Part model, mm, in its own coordinate system. Face numbers are marked on the shaded views. Round coordinates to 2 decimals unless told otherwise and drop trailing zeros. Loops run counter-clockwise (first coordinate to the right, second up) from the corner with the lowest first, then second, coordinate; pieces in that order, holes last. Notation, with made-up numbers: (-39.5, 35.25) -> (13.5, 35.25) arc R4 ccw to (13.5, 41.25) -> close; hole circle Ø6 at (66.25, 44). An arc over 180 degrees is marked (long way). Answer as CSV lines item,"result".
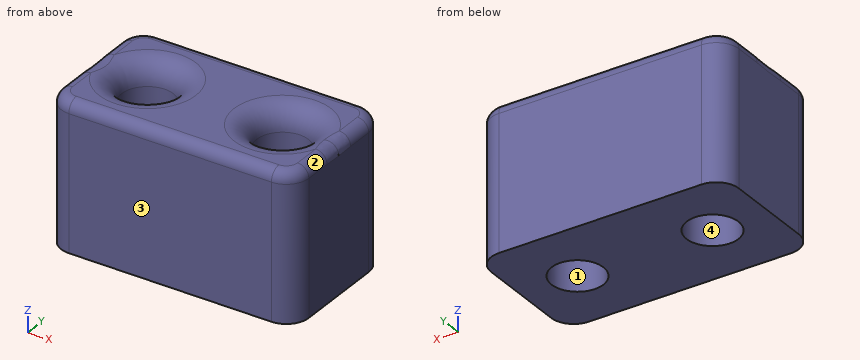
Autodesk Inventor part; units mm, degrees
ref_plane "YZ Plane" through (0, 0, 0) normal (1, 0, 0) x (0, 1, 0)
ref_plane "XZ Plane" through (0, 0, 0) normal (0, 1, 0) x (-1, 0, 0)
ref_plane "XY Plane" through (0, 0, 0) normal (0, 0, 1) x (1, 0, 0)
sketch "Sketch1" plane through (0, 0, 0) normal (0, 0, 1) x (1, 0, 0)
  line L0 (-11, -6) -> (11, -6)
  line L1 (11, -6) -> (11, 6)
  line L2 (11, 6) -> (-11, 6)
  line L3 (-11, 6) -> (-11, -6)
  line L4 (-11, -6) -> (11, 6) construction
  line L5 (11, -6) -> (-11, 6) construction
  circle A0 centre (-6, 0) radius 2.3
  circle A1 centre (6, 0) radius 2.3
  line L6 (-6, 0) -> (0, 0) construction
  line L7 (0, 0) -> (6, 0) construction
  dimension "d0" = 12
  dimension "d1" = 4.6
  dimension "d2" = 12
  dimension "d3" = 5
extrude "Extrusion1" add sketch "Sketch1" along normal blind 13
fillet "Fillet1" radius 2 6 edges at (11, 6, 6.5) (11, -6, 6.5) (-11, 6, 6.5) (-11, -6, 6.5) (-8.3, 0, 13) (3.7, 0, 13)
fillet "Fillet2" radius 1 8 edges at (-10.4142, 5.4142, 13) (-11, 0, 13) (-10.4142, -5.4142, 13) (0, -6, 13) (10.4142, -5.4142, 13) (11, 0, 13) (10.4142, 5.4142, 13) (0, 6, 13)
properties part number "spacer"
Q1. Two-plate mould, pull along X, no slides. Class the marked faces 1, 2, 3 and 4: pulls with the +X half, pulls with the -X half, needs draft (parallel to the pull), parting line crosses it, or undercut.
Geometry results:
face 1,"undercut"
face 2,"pulls with the +X half"
face 3,"needs draft"
face 4,"undercut"
Q2. Saw through at A-A, the plane x = -6. Write the cut outline in (y, z), then the cut area to 3 significant figures.
Geometry results:
outline,"(-6, 0) -> (-2.3, 0) -> (-2.3, 11) arc R2 ccw to (-4.3, 13) -> (-5, 13) arc R1 ccw to (-6, 12) -> close; (2.3, 0) -> (6, 0) -> (6, 12) arc R1 ccw to (5, 13) -> (4.3, 13) arc R2 ccw to (2.3, 11) -> close"
area,"94.1 mm2"
Q3. Drop a flat-ended pin along its axis: P1, Ø6, axis at x = 6, y = 0, coming from the -Z side. Give the stop position or say it passes through.
Geometry results:
P1,"z = 0"
Q4. Saw through at C-C, the plane y = 2. Give the number of separate pieces and of enclosed holes in the cut face, then the cut area to 3 significant figures.
Geometry results:
separate pieces,"3"
enclosed holes,"0"
area,"221 mm2"
Q5. Saw through at B-B, the plane z = 6.75. Write the cut outline in (x, y), then the cut area to 3 significant figures.
Geometry results:
outline,"(-11, -4) arc R2 ccw to (-9, -6) -> (9, -6) arc R2 ccw to (11, -4) -> (11, 4) arc R2 ccw to (9, 6) -> (-9, 6) arc R2 ccw to (-11, 4) -> close; hole circle Ø4.6 at (-6, 0); hole circle Ø4.6 at (6, 0)"
area,"227 mm2"
Q6. Drill centre lines: line 1 along Y through (x, z) = (-6, 5.5); line 2 along Z through (x, y) = (-2.5, -2.25); line 3 along Y through (x, z) = (9.5, 2.75). Where is each one in solid material? Low to high.
Geometry results:
line 1,"-6 to -2.3, 2.3 to 6"
line 2,"0 to 13"
line 3,"-5.94 to 5.94"
